```python
from build123d import *

# Parameters (mm, degrees)
EXTRUDE_DEPTH = 12.6


with BuildPart() as part:
    # Sketch → Extrude (new body, symmetric)
    with BuildSketch(Plane.XZ):
        with BuildLine():
            Line((-219.278359, 26.583984), (-206.078359, 26.583984))
            ThreePointArc((-206.078359, 26.583984), (-205.131957, 26.882383), (-204.527866, 27.669651))
            Line((-204.527866, 27.669651), (-199.861118, 40.491435))
            Line((-199.861118, 40.491435), (-197.061118, 40.491435))
            Line((-197.061118, 40.491435), (-197.061118, 42.891435))
            Line((-197.061118, 42.891435), (-194.261118, 42.891435))
            Line((-194.261118, 42.891435), (-194.534734, 42.139681))
            Line((-194.534734, 42.139681), (-193.031226, 41.592449))
            Line((-193.031226, 41.592449), (-191.663145, 45.351219))
            Line((-191.663145, 45.351219), (-190.535514, 44.940795))
            Line((-190.535514, 44.940795), (-185.747232, 58.096492))
            Line((-185.747232, 58.096492), (-185.747232, 62.096492))
            Line((-185.747232, 62.096492), (-183.831919, 67.35877))
            Line((-183.831919, 67.35877), (-180.231919, 67.35877))
            Line((-180.231919, 67.35877), (-180.231919, 63.75877))
            Line((-180.231919, 63.75877), (-181.6, 60))
            Line((-181.6, 60), (-181.6, 41.2))
            Line((-181.6, 41.2), (-100.8, 41.2))
            Line((-100.8, 41.2), (-100.8, 43.2))
            Line((-100.8, 43.2), (-36, 43.2))
            Line((-36, 43.2), (-36, 48))
            Line((-36, 48), (0, 48))
            Line((0, 48), (0, 0))
            Line((0, 0), (-57.2, 0))
            Line((-57.2, 0), (-57.2, -10.4))
            Line((-57.2, -10.4), (-82.8, -10.4))
            Line((-82.8, -10.4), (-82.8, 3.2))
            Line((-82.8, 3.2), (-93.6, 3.2))
            Line((-93.6, 3.2), (-93.6, 4))
            ThreePointArc((-93.6, 4), (-97.700505, 13.899495), (-107.6, 18))
            Line((-107.6, 18), (-132.428405, 18))
            ThreePointArc((-132.428405, 18), (-140.657398, 15.326238), (-145.743196, 8.326238))
            Line((-145.743196, 8.326238), (-175.232195, -82.431568))
            Line((-175.232195, -82.431568), (-218.032195, -82.431568))
            add(Edge.make_bspline(
                [(-218.032195, -82.431568), (-222.60054, -82.508301), (-229.560425, -71.441643), (-224.432195, -62.431568)],
                knots=[0, 0, 0, 0, 16.552678, 16.552678, 16.552678, 16.552678], degree=3))
            Line((-224.432195, -62.431568), (-203.301282, -17.116179))
            add(Edge.make_bspline(
                [(-203.301282, -17.116179), (-192.874893, -2.614162), (-196.88326, 21.204461), (-218.335348, 22.583984)],
                knots=[0, 0, 0, 0, 54.516173, 54.516173, 54.516173, 54.516173], degree=3))
            Line((-218.335348, 22.583984), (-219.135348, 22.583984))
            ThreePointArc((-219.135348, 22.583984), (-220.266718, 23.052613), (-220.735348, 24.183984))
            Line((-220.735348, 24.183984), (-220.735348, 25.126995))
            ThreePointArc((-220.735348, 25.126995), (-220.308605, 26.157242), (-219.278359, 26.583984))
        make_face()
        with BuildLine():
            Line((-215.122195, -78.431568), (-178.142195, -78.431568))
            Line((-178.142195, -78.431568), (-145.51, 22))
            Line((-145.51, 22), (-87.91, 22))
            Line((-87.91, 22), (-87.91, 10.4))
            Line((-87.91, 10.4), (-78.31, 10.4))
            Line((-78.31, 10.4), (-78.31, 6))
            Line((-78.31, 6), (-4, 6))
            Line((-4, 6), (-4, 36.4))
            Line((-4, 36.4), (-185.2, 36.4))
            Line((-185.2, 36.4), (-190.261898, 22.492549))
            Line((-190.261898, 22.492549), (-191.833618, -4.206153))
            Line((-191.833618, -4.206153), (-199.67605, -18.806652))
            Line((-199.67605, -18.806652), (-220.806963, -64.122041))
            add(Edge.make_bspline(
                [(-215.122195, -78.431568), (-220.482315, -77.450493), (-223.897415, -71.787476), (-220.806963, -64.122041)],
                knots=[0, 0, 0, 0, 15.793542, 15.793542, 15.793542, 15.793542], degree=3))
        make_face(mode=Mode.SUBTRACT)
    extrude(amount=EXTRUDE_DEPTH, both=True)


solid = part.part
```
Check sheet for the modelled part. Datum: model origin and axes. Units: mm. A direction names the side the tool comes from. Round coordinates to 2 decimals unless told otherwise and drop trailing zeros. Order: outer loops, then holes, each group sorted by start corner. A loop starts at its lowest first (then second) coordinate and runs counter-clockwise, first axis right, second up.
1) Section check C-C (z = 55.5). Record the boundary of the cut face in (x, y), and give its area (3 significant figures).
2) Tool access check on faces 4 (the flat face through (-4, 0, 21)), 5 (the cylindrical face through (-140.557, -0.176, 15.398)), 6 (the flat face through (-36, 0, 46)). Record the directions out of +Z, -Z, +X, -X, +Y, -Y that give a thin tool (end or side, any length) a straight path to the whole face; none if there is none.
3) Go/stop test with flat-tipped pins: pin 1 Ø4 at (y, z) = (1.5, 46) entering from -X; pin 2 Ø12.5 at (x, y) = (-14, -4.5) entering from +Z; pin 3 Ø3.5 at (y, z) = (2.5, 9) entering from +X; pin 4 Ø10.5 at (x, y) = (-84, 2.5) entering from +Z. Record where each tip stops, or that it passes through.
4) Scan lines: line 1 (Z direction, x = -111.5, y = 10.5); line 2 (X direction, y = 6.5, z = 20); line 3 (Z direction, x = -90, y = -7.25). Record each from-to range of solid material in increasing order.
5) Section check B-B (x = -140). Record the boundary of the cut face in (y, z).
6) Mould release check, pull along X, two halves, no side actions. Record for faces 1 (the flat face through (-117, 0, 22)), 2 (the flat face through (-213, 0, 26.584)), 3 (the flat face through (-57.2, 0, -5)): +X half, -X half, draft (parallel to the pull), parting line (faces both ways), or undercut.
7) Section check A-A (z = -43). Record the boundary of the cut face in (x, y), and give its area (3 significant figures).
Result:
1. outline: (-186.69, -12.6) - (-181.6, -12.6) - (-181.6, 12.6) - (-186.69, 12.6) - close
1. area: 128 mm2
2. face 4: +Y, -Y
2. face 5: -Z, +Y, -Y
2. face 6: +Z, +Y, -Y
3. pin 1: stops at x = -192.15
3. pin 2: stops at z = 48
3. pin 3: stops at x = 0
3. pin 4: stops at z = 43.2
4. line 1: z = 18 to 22, 36.4 to 41.2
4. line 2: x = -208.72 to -190.41, -146.16 to -87.91, -4 to 0
4. line 3: z = 3.2 to 22, 36.4 to 43.2
5. outline: (-12.6, 15.78) - (12.6, 15.78) - (12.6, 22) - (-12.6, 22) - close; (-12.6, 36.4) - (12.6, 36.4) - (12.6, 41.2) - (-12.6, 41.2) - close
6. face 1: undercut
6. face 2: draft
6. face 3: +X half
7. outline: (-215.37, -12.6) - (-210.96, -12.6) - (-210.96, 12.6) - (-215.37, 12.6) - close; (-166.63, -12.6) - (-162.42, -12.6) - (-162.42, 12.6) - (-166.63, 12.6) - close
7. area: 217 mm2
